from build123d import *

# Parameters (mm, degrees)
ESQUISSE1_W                = 35
ESQUISSE1_H                = 215
BOSS_EXTRU_1_DEPTH         = 6
ESQUISSE2_W                = 18
ESQUISSE2_H                = 6
ENL_V_MAT_EXTRU_1_DEPTH    = 10
ESQUISSE3_W                = 18
ESQUISSE3_H                = 6
ENL_V_MAT_EXTRU_2_DEPTH    = 218.912826607
ESQUISSE4_W                = 11
ESQUISSE4_H                = 48.05464589
ENL_V_MAT_EXTRU_3_DEPTH    = 218.912826607
ESQUISSE5_R                = 2.5
ENL_V_MAT_EXTRU_4_DEPTH    = 10
R_P_TITION_LIN_AIRE1_COUNT = 2
R_P_TITION_LIN_AIRE1_PITCH = 29


with BuildPart() as part:
    # Esquisse1 → Boss.-Extru.1 (new body)
    with BuildSketch(Plane.XY):
        with Locations((17.5, 107.5)):
            Rectangle(ESQUISSE1_W, ESQUISSE1_H)
    extrude(amount=BOSS_EXTRU_1_DEPTH)

    # Esquisse2 → Enlèv. mat.-Extru.1 (cut)
    with BuildSketch(Plane(origin=(0, 215, 0), x_dir=(1, 0, 0), z_dir=(0, 1, 0))):
        with Locations((18, -3)):
            Rectangle(ESQUISSE2_W, ESQUISSE2_H)
    extrude(amount=-ENL_V_MAT_EXTRU_1_DEPTH, mode=Mode.SUBTRACT)

    # Esquisse3 → Enlèv. mat.-Extru.2 (cut, through all)
    with BuildSketch(Plane.XY.offset(6)):
        with Locations((18, 178)):
            Rectangle(ESQUISSE3_W, ESQUISSE3_H)
    extrude(amount=-ENL_V_MAT_EXTRU_2_DEPTH, mode=Mode.SUBTRACT)

    # Esquisse4 → Enlèv. mat.-Extru.3 (cut, through all)
    with BuildSketch(Plane(origin=(0, 0, 0), x_dir=(-1, 0, 0), z_dir=(0, 0, -1))):
        with Locations((-5.5, 144.027326709)):
            Rectangle(ESQUISSE4_W, ESQUISSE4_H)
    extrude(amount=-ENL_V_MAT_EXTRU_3_DEPTH, mode=Mode.SUBTRACT)

    # Esquisse5 → Enlèv. mat.-Extru.4 (cut)
    with BuildSketch(Plane(origin=(0, 215, 0), x_dir=(1, 0, 0), z_dir=(0, 1, 0))):
        with Locations(Location((3, -3, 0), (0, 0, 270))):
            Circle(ESQUISSE5_R)
    enl_v_mat_extru_4 = extrude(amount=-ENL_V_MAT_EXTRU_4_DEPTH, mode=Mode.SUBTRACT)

    # Répétition linéaire1: Enlèv. mat.-Extru.4 ×2
    with Locations(*[(i * R_P_TITION_LIN_AIRE1_PITCH, 0, 0) for i in range(1, R_P_TITION_LIN_AIRE1_COUNT)]):
        add(enl_v_mat_extru_4, mode=Mode.SUBTRACT)


solid = part.part
Check sheet for the modelled part. Datum: model origin and axes. Units: mm. A direction names the side the tool comes from. Coordinates: 2 decimals unless noted, no trailing zeros. Write each loop counter-clockwise with the first axis right and the second up, starting at its lowest first coordinate (ties: lowest second). Pieces come first, ordered by that corner, then holes.
Item 1: Cross-section at C-C on x = 22. Record the boundary of the cut face in (y, z), then the cut area to 3 significant figures.
Numbers:
outline: (0, 0) - (175, 0) - (175, 6) - (0, 6) - close; (181, 0) - (205, 0) - (205, 6) - (181, 6) - close
area: 1,190 mm2
Item 2: Access from +Z, -Z, +X, -X, +Y, -Y to the whole of each face (thin tool, end or side, straight path). Record for faces 1 (the face through (9, 178, 3)), 2 (the face through (27, 210, 3)), 3 (the face through (0.56, 210.07, 2.46)), 4 (the face through (6, 168.055, 3)), 5 (the face through (29, 215, 3)).
Numbers:
face 1: +Z, -Z
face 2: +Z, -Z, +Y
face 3: +Y
face 4: +Z, -Z, -X
face 5: +Z, -Z, +X, -X, +Y
Item 3: Mould release check, pull along X, two halves, no side actions. Record for faces 6 (the face through (6, 215, 3)), 7 (the face through (35, 106, 3)), 8 (the face through (9, 210, 3)), 9 (the face through (11, 144, 3)): released by +X, released by -X, zero draft, split by the parting line, or undercut.
Numbers:
face 6: zero draft
face 7: released by +X
face 8: undercut
face 9: released by -X
Item 4: Depth check by flat-ended pin: pin 1 Ø1 at (x, z) = (31, 2.5) entering from -Y; pin 2 Ø1.5 at (x, z) = (31.5, 2) entering from +Y; pin 3 Ø1.8 at (y, z) = (135.5, 1.5) entering from -X. Enter the tip coordinate at first touch or a pass-through.
Numbers:
pin 1: stops at y = 0
pin 2: stops at y = 205
pin 3: stops at x = 11
Item 5: Scan lines: probe 1 along X at (y, z) = (210, 3); probe 2 along Y at (x, z) = (7.5, 4); probe 3 along Y at (x, z) = (3.5, 1.95). Record each from-to range of solid material in increasing order.
Numbers:
probe 1: x = 0 to 0.5, 5.5 to 9, 27 to 29.5, 34.5 to 35
probe 2: y = 0 to 120, 168.05 to 215
probe 3: y = 0 to 120, 168.05 to 205
Item 6: Cross-section at A-A on x = 3. Record the boundary of the cut face in (y, z), then the cut area to 3 significant figures.
Numbers:
outline: (0, 0) - (120, 0) - (120, 6) - (0, 6) - close; (168.05, 0) - (215, 0) - (215, 0.5) - (205, 0.5) - (205, 5.5) - (215, 5.5) - (215, 6) - (168.05, 6) - close
area: 952 mm2
Item 7: Cross-section at D-D on x = 32. Record the boundary of the cut face in (y, z).
Numbers:
outline: (0, 0) - (215, 0) - (215, 0.5) - (205, 0.5) - (205, 5.5) - (215, 5.5) - (215, 6) - (0, 6) - close
Item 8: Cross-section at B-B on z = 3. Record the boundary of the cut face in (x, y).
Numbers:
outline: (0, 0) - (35, 0) - (35, 215) - (34.5, 215) - (34.5, 205) - (29.5, 205) - (29.5, 215) - (27, 215) - (27, 205) - (9, 205) - (9, 215) - (5.5, 215) - (5.5, 205) - (0.5, 205) - (0.5, 215) - (0, 215) - (0, 168.05) - (11, 168.05) - (11, 120) - (0, 120) - close; hole (9, 175) - (27, 175) - (27, 181) - (9, 181) - close
